from build123d import *

# Parameters (mm, degrees)
BOSS_EXTRUDE1_DEPTH = 1.524


with BuildPart() as part:
    # Sketch1 → Boss-Extrude1 (new body)
    with BuildSketch(Plane.XY):
        with BuildLine():
            Line((0, -1.964327556), (-1.524, -1.964327556))
            Line((-1.524, -1.964327556), (-1.524, 0.132092651))
            Line((-1.524, 0.132092651), (0, 0.132092651))
            Line((0, 0.132092651), (0, 1.699735594))
            Line((0, 1.699735594), (-1.524, 1.699735594))
            Line((-1.524, 1.699735594), (-1.524, 7.30837055))
            Line((-1.524, 7.30837055), (-1.524, 10.365124178))
            Line((-1.524, 10.365124178), (-6.782878703, 10.365124178))
            ThreePointArc((-6.782878703, 10.365124178), (-6.783116279, 6.194251187), (-5.086577691, 2.384009936))
            ThreePointArc((-5.086577691, 2.384009936), (-4.509773665, -0.889665066), (-5.086577691, -4.163340068))
            ThreePointArc((-5.086577691, -4.163340068), (-7.205112449, -8.282791607), (-6.536296983, -12.866540768))
            Line((-6.536296983, -12.866540768), (0.285426682, -12.866540768))
            Line((0.285426682, -12.866540768), (0.285426682, -14.508842733))
            Line((0.285426682, -14.508842733), (-5.954978709, -14.508842733))
            ThreePointArc((-5.954978709, -14.508842733), (-4.027344351, -16.471916174), (-1.321752383, -16.971119191))
            ThreePointArc((-1.321752383, -16.971119191), (2.319118957, -15.86929322), (5.959990297, -16.971119191))
            ThreePointArc((5.959990297, -16.971119191), (10.949556437, -14.851489508), (14.666489015, -10.905223871))
            ThreePointArc((14.666489015, -10.905223871), (10.922843112, -12.5189914), (6.861028282, -12.866540768))
            ThreePointArc((6.861028282, -12.866540768), (1.349866502, -9.785380814), (-1.524, -4.163340068))
            Line((-1.524, -4.163340068), (0, -4.163340068))
            Line((0, -4.163340068), (0, -1.964327556))
        make_face()
    extrude(amount=BOSS_EXTRUDE1_DEPTH)


solid = part.part
Part model, mm, in its own coordinate system. A direction names the side the tool comes from. Round coordinates to 2 decimals unless told otherwise and drop trailing zeros. Write each loop counter-clockwise with the first axis right and the second up, starting at its lowest first coordinate (ties: lowest second). Pieces come first, ordered by that corner, then holes. Notation, with made-up numbers: M -4,11 L 29,11 A30 cw 29,48 Z; hole C 38.5,19 d8. An arc over 180 degrees is marked long. Return JSON: item names as keys, results as strings. Group by question number.
(1) Drill centre lines: probe 1 along Y at (x, z) = (-1.75, 0.75); probe 2 along Y at (x, z) = (-3, 0.9); probe 3 along X at (y, z) = (7.25, 1.05). Where is each one in solid material? Low to high.
(2) Pin check, flat tips, straight feed: pin 1 Ø0.8 at (x, z) = (-1, 1) entering from -Y; pin 2 Ø0.8 at (x, z) = (-1, 0.5) entering from +Y; pin 3 Ø0.8 at (y, z) = (5, 0.5) entering from +X. Stop position of each tip, or through.
(3) Two-plate mould, pull along X, no slides. Class faces 1 (the face through (-1.524, -1, 1)), 2 (the face through (1.41, -9.85, 0.75)), 3 (the face through (-1.3, -6.3, 1.524)): +X half, -X half, draft (parallel to the pull), parting line (faces both ways), or undercut.
(4) Which spindle directions (+Z, -Z, +X, -X, +Y, -Y) get a long thin tool onto all of the face, cutting with end or side? Do faces 4 (the face through (10.887, -14.895, 0.751)), 5 (the face through (-1.524, 6, 1)), 6 (the face through (0.285, -14, 1)), 7 (the face through (-1, -4.163, 1)). Say none if no direction does.
(5) Saw through at C-C on z = 1.2. Write the cut outline in (x, y), then the cut area to 3 significant figures.
(6) Saw through at A-A on x = -2.5. Write the cut outline in (y, z), then the cut area to 3 significant figures.
(7) Saw through at B-B on y = -12. Write the cut outline in (x, z).
(8) Saw through at D-D on x = 1.75. Write the cut outline in (y, z), then the cut area to 3 significant figures.
Returned:
{
 "1": {"probe 1": "-17 to -14.51, -12.87 to 10.37", "probe 2": "-16.87 to -14.51, -12.87 to 10.37", "probe 3": "-6.95 to -1.52"},
 "2": {"pin 1": "y = -16.98", "pin 2": "y = 1.7", "pin 3": "x = -1.52"},
 "3": {"face 1": "+X half", "face 2": "undercut", "face 3": "draft"},
 "4": {"face 4": "+Z, -Z, +X, -Y", "face 5": "+Z, -Z, +X, +Y", "face 6": "+Z, -Z, -X", "face 7": "+Z, -Z, +X"},
 "5": {"outline": "M -6.78,10.37 A10.03 ccw -5.09,2.38 A9.58 cw -5.09,-4.16 A7.59 ccw -6.54,-12.87 L 0.29,-12.87 L 0.29,-14.51 L -5.95,-14.51 A4.57 ccw -1.32,-16.97 A6.57 cw 5.96,-16.97 A13.2 ccw 14.67,-10.91 A12.73 cw 6.86,-12.87 A10.89 cw -1.52,-4.16 L 0,-4.16 L 0,-1.96 L -1.52,-1.96 L -1.52,0.13 L 0,0.13 L 0,1.7 L -1.52,1.7 L -1.52,10.37 Z", "area": "186 mm²"},
 "6": {"outline": "M -16.96,0 L -14.51,0 L -14.51,1.52 L -16.96,1.52 Z; M -12.87,0 L 10.37,0 L 10.37,1.52 L -12.87,1.52 Z", "area": "39.1 mm²"},
 "7": {"outline": "M -6.9,0 L 4.38,0 L 4.38,1.52 L -6.9,1.52 Z; M 12.53,0 L 13.92,0 L 13.92,1.52 L 12.53,1.52 Z"},
 "8": {"outline": "M -15.89,0 L -10.18,0 L -10.18,1.52 L -15.89,1.52 Z", "area": "8.71 mm²"}
}
